The model under review builds one solid part; all positions refer to its coordinate system, in mm. Face numbers are marked on the shaded views. A direction names the side the tool comes from. Round coordinates to 2 decimals unless told otherwise and drop trailing zeros. Write each loop counter-clockwise with the first axis right and the second up, starting at its lowest first coordinate (ties: lowest second). Pieces come first, ordered by that corner, then holes. Notation, with made-up numbers: (39.25, 35) - (62.25, 35) arc R22 ccw to (62.25, 60) - close; hole circle Ø6 at (0, 9). An arc over 180 degrees is marked (long way). Return JSON: item names as keys, results as strings.
from build123d import *

# Parameters (mm, degrees)
BOSS_EXTRU_1_DEPTH           = 11.6
ESQUISSE2_R                  = 10
BOSS_EXTRU_2_DEPTH           = 9
ENL_V_MAT_EXTRU_1_DEPTH      = 37.999763513
ENL_V_MAT_EXTRU_1_DEPTH_BACK = 37.999763513
ESQUISSE3_R                  = 1.6
ENL_V_MAT_EXTRU_2_DEPTH      = 41.252111746
ENL_V_MAT_EXTRU_2_DEPTH_BACK = 41.252111746
CHANFREIN1_SIZE              = 2
ESQUISSE7_R                  = 11
ESQUISSE7_R_2                = 1.6
BOSS_EXTRU_3_DEPTH           = 6
ENL_V_MAT_EXTRU_3_DEPTH      = 10
R_P_TITION_CIRCULAIRE1_COUNT = 2


with BuildPart() as part:
    # Esquisse1 → Boss.-Extru.1 (new body)
    with BuildSketch(Plane(origin=(0, 0, 0), x_dir=(1, 0, 0), z_dir=(0, 1, 0))):
        Polygon((7.5, 27.85), (-7.5, 27.85), (-7.5, 10.85), (-13, 5), (-13, -5), (-7.5, -10.85), (-7.5, -27.85), (7.5, -27.85), (7.5, -10.85), (13, -5), (13, 5), (7.5, 10.85), align=None)
    extrude(amount=BOSS_EXTRU_1_DEPTH)

    # Esquisse2 → Boss.-Extru.2 (add)
    with BuildSketch(Plane(origin=(0, 11.6, 0), x_dir=(1, 0, 0), z_dir=(0, 1, 0))):
        with Locations(Location((0, 0, 0), (0, 0, 270))):
            Circle(ESQUISSE2_R)
    extrude(amount=BOSS_EXTRU_2_DEPTH)

    # Esquisse3 → Enlèv. mat.-Extru.1 (cut, two sides: drawn at the far end of the back side and taken through both)
    with BuildSketch(Plane.XZ.offset(-ENL_V_MAT_EXTRU_1_DEPTH_BACK)):
        with Locations(Location((0, 6, 0), (0, 0, 270))):
            Circle(ESQUISSE3_R)
        with Locations(Location((0, -6, 0), (0, 0, 270))):
            Circle(ESQUISSE3_R)
    extrude(amount=ENL_V_MAT_EXTRU_1_DEPTH + ENL_V_MAT_EXTRU_1_DEPTH_BACK, mode=Mode.SUBTRACT)

    # Esquisse6 → Enlèv. mat.-Extru.2 (cut, two sides: drawn at the far end of the back side and taken through both)
    with BuildSketch(Plane.ZY.offset(7.5).offset(-ENL_V_MAT_EXTRU_2_DEPTH_BACK)):
        Polygon((16.1, 6.810362971), (17.85, 7.820725942), (19.6, 6.810362971), (19.6, 4.789637029), (17.85, 3.779274058), (16.1, 4.789637029), align=None)
        Polygon((-17.85, 7.820725942), (-19.6, 6.810362971), (-19.6, 4.789637029), (-17.85, 3.779274058), (-16.1, 4.789637029), (-16.1, 6.810362971), align=None)
    extrude(amount=ENL_V_MAT_EXTRU_2_DEPTH + ENL_V_MAT_EXTRU_2_DEPTH_BACK, mode=Mode.SUBTRACT)

    # Chanfrein1
    chanfrein1_edges = [part.edges().sort_by_distance(p)[0] for p in [
        (0, 11.6, 27.85),
        (0, 11.6, -27.85),
    ]]
    chamfer(chanfrein1_edges, length=CHANFREIN1_SIZE)

    # Esquisse7 → Boss.-Extru.3 (add)
    with BuildSketch(Plane(origin=(0, 11.6, 0), x_dir=(1, 0, 0), z_dir=(0, 1, 0))):
        with Locations(Location((0, 0, 0), (0, 0, 90))):
            Circle(ESQUISSE7_R)
        with Locations(Location((0, 6, 0), (0, 0, 90))):
            Circle(ESQUISSE7_R_2, mode=Mode.SUBTRACT)
        with Locations(Location((0, -6, 0), (0, 0, 90))):
            Circle(ESQUISSE7_R_2, mode=Mode.SUBTRACT)
    extrude(amount=BOSS_EXTRU_3_DEPTH)

    # Esquisse8 → Enlèv. mat.-Extru.3 (cut)
    with BuildSketch(Plane.XZ):
        Polygon((0, 9.233161507), (-2.8, 7.616580754), (-2.8, 4.383419246), (0, 2.766838493), (2.8, 4.383419246), (2.8, 7.616580754), align=None)
    enl_v_mat_extru_3 = extrude(amount=-ENL_V_MAT_EXTRU_3_DEPTH, mode=Mode.SUBTRACT)

    # Répétition circulaire1: Enlèv. mat.-Extru.3 ×2 about axis
    r_p_tition_circulaire1_axis = Axis((0, 0, 0), (0, 1, 0))
    for i in range(1, R_P_TITION_CIRCULAIRE1_COUNT):
        add(enl_v_mat_extru_3.rotate(r_p_tition_circulaire1_axis, i * 360 / R_P_TITION_CIRCULAIRE1_COUNT), mode=Mode.SUBTRACT)


solid = part.part
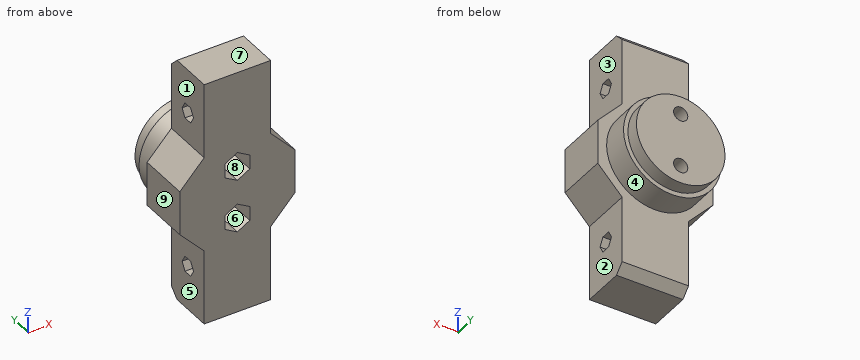
(1) Wall thickness on line 1 (Z direction, x = 0, y = 18.75); line 2 (Z direction, x = 2.75, y = 6.5); line 3 (Z direction, x = 0.75, y = 15.25): over which ranges is each line inside the solid? List them lowest first.
Filled in:
{"line 1": "z = -10 to -7.6, -4.4 to 4.4, 7.6 to 10", "line 2": "z = -27.85 to -19.6, -16.1 to -7.65, -4.35 to 4.35, 7.65 to 16.1, 19.6 to 27.85", "line 3": "z = -10.97 to -7.41, -4.59 to 4.59, 7.41 to 10.97"}
(2) Add section A-A (y = 6.25). Give the number of separate pieces and of enclosed holes in the cut face, plus the area to 3 significant figures.
Filled in:
{"separate pieces": "3", "enclosed holes": "2", "area": "851 mm2"}
(3) Add section B-B (y = 3). Write out the cut boundary in (x, z).
Filled in:
{"outline": "(-13, -5) - (-7.5, -10.85) - (-7.5, -27.85) - (7.5, -27.85) - (7.5, -10.85) - (13, -5) - (13, 5) - (7.5, 10.85) - (7.5, 27.85) - (-7.5, 27.85) - (-7.5, 10.85) - (-13, 5) - close; hole (-2.8, -7.62) - (0, -9.23) - (2.8, -7.62) - (2.8, -4.38) - (0, -2.77) - (-2.8, -4.38) - close; hole (-2.8, 4.38) - (0, 2.77) - (2.8, 4.38) - (2.8, 7.62) - (0, 9.23) - (-2.8, 7.62) - close"}
(4) For the marked faces 1, 2, 3, 4 and 5, list the 3-axis set-ups (+Z, -Z, +X, -X, +Y, -Y) from which the entire face can be reached by the end or side of a thin tool; tool diameter is ignored.
Filled in:
{"face 1": "+Z, -X, +Y, -Y", "face 2": "-Z, +X, +Y, -Y", "face 3": "+Z, +X, +Y, -Y", "face 4": "+Y", "face 5": "-Z, -X, +Y, -Y"}
(5) Clearance check with flat-ended pins moving along their axes: pin 1 Ø9.5 at (y, z) = (5.5, -17.5) entering from +X; pin 2 Ø3 at (y, z) = (11.5, -21.5) entering from -X; pin 3 Ø2.5 at (y, z) = (7, 6) entering from +X; pin 4 Ø2.5 at (y, z) = (5.5, -6.5) entering from -X. State where each tip first meets the part, or that it passes through.
Filled in:
{"pin 1": "stops at x = 7.5", "pin 2": "stops at x = -7.5", "pin 3": "stops at x = 13", "pin 4": "stops at x = -12.76"}
(6) Add section D-D (x = -6.75). Write out the cut boundary in (y, z).
Filled in:
{"outline": "(0, -27.85) - (9.6, -27.85) - (11.6, -25.85) - (11.6, -8.69) - (17.6, -8.69) - (17.6, -7.38) - (20.6, -7.38) - (20.6, 7.38) - (17.6, 7.38) - (17.6, 8.69) - (11.6, 8.69) - (11.6, 25.85) - (9.6, 27.85) - (0, 27.85) - close; hole (3.78, -17.85) - (4.79, -19.6) - (6.81, -19.6) - (7.82, -17.85) - (6.81, -16.1) - (4.79, -16.1) - close; hole (3.78, 17.85) - (4.79, 16.1) - (6.81, 16.1) - (7.82, 17.85) - (6.81, 19.6) - (4.79, 19.6) - close"}
(7) Mouldability with a two-part tool opening along Z and no side actions: class the marked faces 6, 7, 8 and 9 as released by +Z, released by -Z, zero draft, split by the parting line, or undercut.
Filled in:
{"face 6": "undercut", "face 7": "released by +Z", "face 8": "undercut", "face 9": "zero draft"}
(8) Add section C-C (z = -19). Write out the cut boundary in (x, y).
Filled in:
{"outline": "(-7.5, 0) - (7.5, 0) - (7.5, 4.44) - (-7.5, 4.44) - close; (-7.5, 7.16) - (7.5, 7.16) - (7.5, 11.6) - (-7.5, 11.6) - close"}
